Input: part model. Units: mm. Frame: model coordinates. Face numbers are marked on the shaded views. A direction names the side the tool comes from. Round coordinates to 2 decimals unless told otherwise and drop trailing zeros. Loops run counter-clockwise (first coordinate to the right, second up) from the corner with the lowest first, then second, coordinate; pieces in that order, holes last. Notation, with made-up numbers: (27.25, -26.5) -> (45.25, -26.5) arc R10 cw to (45.25, -18.5) -> close; hole circle Ø6 at (76.5, 65). An arc over 180 degrees is marked (long way). One line per question, with ' | ' between items. Start each with the question number.
Q1. Cut plane C-C on y = 4.5. Return loops of the section in (x, z).
Q2. Cut plane D-D on x = 5.5. Return loops of the section in (y, z).
Q3. Access query for the marked faces 1 and 2. Directions: +Z, -Z, +X, -X, +Y, -Y. A direction counts if a zero-diameter tool reaches every point of the face in a straight line with its end or side. Return the directions, or none.
Q4. Mould query, pull axis Y, two halves, no side actions, for the marked faces 3, 4 and 5. Classes: pulls with the +Y half, pulls with the -Y half, needs draft (parallel to the pull), parting line crosses it, or undercut.
Q5. Material intervals for L1, parallel to X at y = 0.9, z = 5.8; L2, parallel to Y at x = 39, z = 6; L3, parallel to Z at x = 30.5, y = 1.5, sorted ascending.
Q6. Contact query for a flat-ended pin moving along its axis: P1, Ø5, axis at x = 36.5, z = 5.8, coming from the +Y side. Output: stop coordinate, or through.
Q7. Cut plane A-A on x = 27.5. Return loops of the section in (y, z).
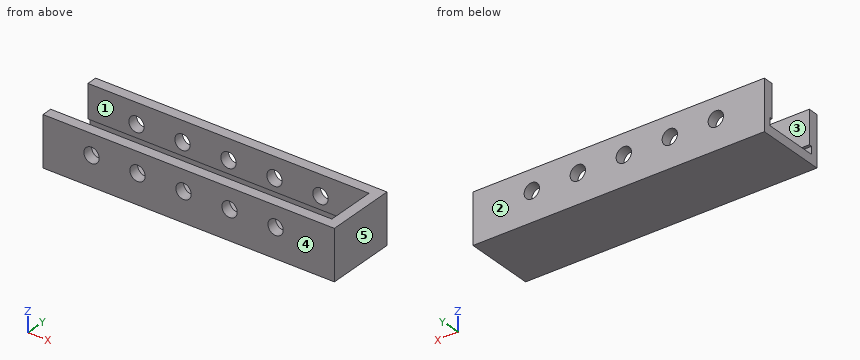
from build123d import *

# Parameters (mm, degrees)
SKETCH_1_W          = 57
SKETCH_1_H          = 13.7
EXTRUDE_1_DEPTH     = 9.8
SKETCH_2_W          = 55
SKETCH_2_H          = 9.7
CUT_EXTRUDE_1_DEPTH = 8
SKETCH_3_W          = 54.972087022
SKETCH_3_H          = 0.6
CUT_EXTRUDE_2_DEPTH = 1.5
SKETCH_4_R          = 1.5
CUT_EXTRUDE_3_DEPTH = 14


with BuildPart() as part:
    # Эскиз1 → Бобышка-Вытянуть1 (new body)
    with BuildSketch(Plane.XY):
        with Locations((28.5, 6.85)):
            Rectangle(SKETCH_1_W, SKETCH_1_H)
    extrude(amount=EXTRUDE_1_DEPTH)

    # Эскиз2 → Вырез-Вытянуть1 (cut)
    with BuildSketch(Plane.XY.offset(9.8)):
        with Locations((27.5, 6.85)):
            Rectangle(SKETCH_2_W, SKETCH_2_H)
    extrude(amount=-CUT_EXTRUDE_1_DEPTH, mode=Mode.SUBTRACT)

    # Эскиз3 → Вырез-Вытянуть2 (cut)
    with BuildSketch(Plane.XY.offset(1.8)):
        with Locations((27.486043511, 12)):
            Rectangle(SKETCH_3_W, SKETCH_3_H)
        with Locations((27.486043511, 1.7)):
            Rectangle(SKETCH_3_W, SKETCH_3_H)
    extrude(amount=CUT_EXTRUDE_2_DEPTH, mode=Mode.SUBTRACT)

    # Эскиз4 → Вырез-Вытянуть3 (cut)
    with BuildSketch(Plane(origin=(0, 13.7, 0), x_dir=(1, 0, 0), z_dir=(0, 1, 0))):
        with Locations(Location((45.5, -5.8, 0), (0, 0, 270))):
            Circle(SKETCH_4_R)
        with Locations(Location((36.5, -5.8, 0), (0, 0, 270))):
            Circle(SKETCH_4_R)
        with Locations(Location((27.5, -5.8, 0), (0, 0, 270))):
            Circle(SKETCH_4_R)
        with Locations(Location((18.5, -5.8, 0), (0, 0, 270))):
            Circle(SKETCH_4_R)
        with Locations(Location((9.5, -5.8, 0), (0, 0, 270))):
            Circle(SKETCH_4_R)
    extrude(amount=-CUT_EXTRUDE_3_DEPTH, mode=Mode.SUBTRACT)


solid = part.part
Results:
1) outline: (0, 0) -> (57, 0) -> (57, 9.8) -> (55, 9.8) -> (55, 1.8) -> (0, 1.8) -> close
2) outline: (0, 0) -> (13.7, 0) -> (13.7, 9.8) -> (11.7, 9.8) -> (11.7, 3.3) -> (12.3, 3.3) -> (12.3, 1.8) -> (1.4, 1.8) -> (1.4, 3.3) -> (2, 3.3) -> (2, 9.8) -> (0, 9.8) -> close
3) face 1: +Z, -X | face 2: +Z, -Z, +X, -X, +Y
4) face 3: undercut | face 4: pulls with the -Y half | face 5: needs draft
5) L1: 0 to 8, 11 to 17, 20 to 26, 29 to 35, 38 to 44, 47 to 57 | L2: 0 to 2, 11.7 to 13.7 | L3: 0 to 1.8, 3.3 to 9.8
6) P1: y = 13.7
7) outline: (0, 0) -> (13.7, 0) -> (13.7, 4.3) -> (11.7, 4.3) -> (11.7, 3.3) -> (12.3, 3.3) -> (12.3, 1.8) -> (1.4, 1.8) -> (1.4, 3.3) -> (2, 3.3) -> (2, 4.3) -> (0, 4.3) -> close; (0, 7.3) -> (2, 7.3) -> (2, 9.8) -> (0, 9.8) -> close; (11.7, 7.3) -> (13.7, 7.3) -> (13.7, 9.8) -> (11.7, 9.8) -> close
